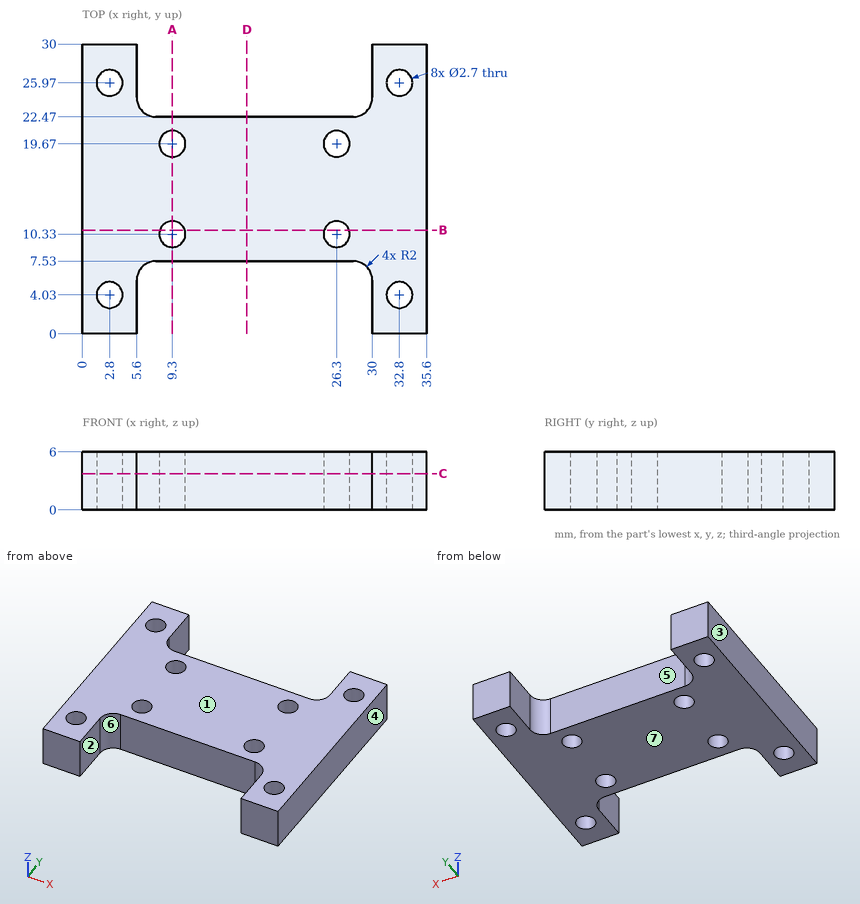
Can you work these out from the drawing? Everything is in mm from the part's minimum corner. A direction names the side the tool comes from. Round coordinates to 2 decimals unless told otherwise and drop trailing zeros. Loops run counter-clockwise (first coordinate to the right, second up) from the corner with the lowest first, then second, coordinate; pieces in that order, holes last. Notation, with made-up numbers: M 3,75 L 49,75 A17 cw 49,105 Z; hole C 45,34 d8. An arc over 180 degrees is marked long. Answer in a Markdown table with one row per item.
1. I'm going to push a flat-ended pin straight in: pin 1 Ø4 at (x, y) = (9, 15.5) entering from -Z. Where does the tip first touch, or does it pass through?
Established:
| item | result |
|---|---|
| pin 1 | z = 0 |
2. On a 3-axis mill with a long thin cutter (end or side, diameter ignored), from which of +Z, -Z, +X, -X, +Y, -Y can I reach the whole of each face in a straight line? I mean the marked faces 5, 6 and 7. Say none if no direction works.
Established:
| item | result |
|---|---|
| face 5 | +Z, -Z, +Y |
| face 6 | +Z, -Z, -Y |
| face 7 | -Z, +X, -X, +Y, -Y |
3. If we section it at C-C, the plane z = 3.75: Give the number of separate pieces and of enclosed holes in the cut face, plus the area to 3 significant figures.
Established:
| item | result |
|---|---|
| separate pieces | 1 |
| enclosed holes | 8 |
| area | 658 mm² |
4. Please list where these lines run through material, in increasing order: line 1 (Y direction, x = 2.8, z = 2.35); line 2 (Y direction, x = 26.3, z = 3.45); line 3 (X direction, y = 27.5, z = 2.65). Write a range as from..to.
Established:
| item | result |
|---|---|
| line 1 | 0..2.68, 5.38..24.62, 27.32..30 |
| line 2 | 7.53..8.98, 11.68..18.32, 21.02..22.47 |
| line 3 | 0..5.6, 30..35.6 |
5. Thinking about a two-plate mould opening in X: for the marked faces 1, 2, 3 and 4, which applies, pulls with the +X half, pulls with the -X half, needs draft (parallel to the pull), parting line crosses it, or undercut?
Established:
| item | result |
|---|---|
| face 1 | needs draft |
| face 2 | undercut |
| face 3 | pulls with the -X half |
| face 4 | pulls with the +X half |
6. If we section it at D-D, the plane x = 17: Please give me the cut outline in (y, z).
Established:
| item | result |
|---|---|
| outline | M 7.53,0 L 22.47,0 L 22.47,6 L 7.53,6 Z |
7. If we section it at B-B, the plane y = 10.75: Please give me the cut outline in (x, z), plus the area to 3 significant figures.
Established:
| item | result |
|---|---|
| outline | M 0,0 L 8.02,0 L 8.02,6 L 0,6 Z; M 10.58,0 L 25.02,0 L 25.02,6 L 10.58,6 Z; M 27.58,0 L 35.6,0 L 35.6,6 L 27.58,6 Z |
| area | 183 mm² |
8. If we section it at A-A, the plane x = 9.3: Please give me the cut outline in (y, z).
Established:
| item | result |
|---|---|
| outline | M 7.53,0 L 8.98,0 L 8.98,6 L 7.53,6 Z; M 11.68,0 L 18.32,0 L 18.32,6 L 11.68,6 Z; M 21.02,0 L 22.47,0 L 22.47,6 L 21.02,6 Z |
